Can you work these out from the model? Positions are in its coordinate system, mm. A direction names the side the tool comes from. Coordinates: 2 decimals unless noted, no trailing zeros. Loops run counter-clockwise (first coordinate to the right, second up) from the corner with the lowest first, then second, coordinate; pieces in that order, holes last. Notation, with made-up numbers: (-15, 53.5) -> (22, 53.5) arc R4 cw to (22, 58.5) -> close; hole circle Ø5 at (78.25, -26.75). An arc over 180 degrees is marked (long way). Use one line per item in the form item = value. Start each with the question number.
(1) I'm going to push flat-ended pins straight in: pin 1 (17 mm diameter, centred on x = 60, y = 50.5, fed in from +Z); pin 2 (3 mm diameter, centred on x = 55, y = 30.5, fed in from +Z); pin 3 (1 mm diameter, centred on y = 39.5, z = 3, fed in from -X); pin 4 (0.9 mm diameter, centred on y = 35.5, z = 2.5, fed in from +X). Where does each tip first touch, or does it pass through?
(2) On a 3-axis mill with a long thin cutter (end or side, diameter ignored), from which of +Z, -Z, +X, -X, +Y, -Y can I reach the whole of each face in a straight line? I mean faces 1 (the flat face through (31.483, 58, 1)), 2 (the flat face through (94.183, 40, 3)), 3 (the flat face through (63.267, 43.688, 2.521)), 4 (the flat face through (31.483, 39, 3)). Say none if no direction works.
(3) Imagine slicing it at A-A (y = 62.5). List the corners of the cut face in (x, z) for me, plus the area to 3 significant figures.
(4) Imagine slicing it at D-D (y = 18.5). List the corners of the cut face in (x, z) for me.
(5) Imagine slicing it at B-B (x = 87.5). List the corners of the cut face in (y, z) for me.
(6) Imagine slicing it at C-C (z = 3.3). List the corners of the cut face in (x, y) for me, plus the area to 3 significant figures.
(7) I need wall thicknesses on line 1 (Y direction, x = 70, z = 0.8); line 2 (Y direction, x = 55, z = 1.4); line 3 (X direction, y = 48, z = 1.55). Which ranges of each line are inside material? Lowest first, please. Write a range as [from, to].
(8) Thinking about a two-plate mould opening in Y: for faces 5 (the flat face through (62, 68.292, 1)), 6 (the flat face through (96.083, 40, 1)), 7 (the flat face through (62.4, 66.392, 1.2)), which applies, released by +Y, released by -Y, zero draft, split by the parting line, or undercut?
Autodesk Fusion 360 part; units mm, degrees
sketch "Schizzo1" plane through (0, 0, 0) normal (0, 0, 1) x (1, 0, 0)
  line L0 (29.4832, 68.3919) -> (96.1832, 68.3919) construction
  line L1 (96.1832, 68.3919) -> (96.1832, 10.6919) construction
  line L2 (96.1832, 10.6919) -> (29.4832, 10.6919) construction
  line L3 (29.4832, 10.6919) -> (29.4832, 68.3919) construction
  line L4 (96.0832, 10.7919) -> (29.5832, 10.7919)
  line L5 (29.5832, 10.7919) -> (29.5832, 68.2919)
  line L6 (29.5832, 68.2919) -> (96.0832, 68.2919)
  line L7 (96.0832, 68.2919) -> (96.0832, 10.7919)
  line L8 (94.1832, 12.6919) -> (31.4832, 12.6919)
  line L9 (31.4832, 12.6919) -> (31.4832, 66.3919)
  line L10 (31.4832, 66.3919) -> (94.1832, 66.3919)
  line L11 (94.1832, 66.3919) -> (94.1832, 12.6919)
  line L12 (31.4832, 66.3919) -> (57.4832, 66.3919)
  line L13 (57.4832, 66.3919) -> (57.4832, 56.3919)
  line L14 (57.4832, 56.3919) -> (31.4832, 56.3919)
  line L15 (31.4832, 56.3919) -> (31.4832, 66.3919)
  line L16 (65.4832, 66.3919) -> (91.4832, 66.3919)
  line L17 (91.4832, 56.3919) -> (65.4832, 56.3919)
  line L18 (91.4832, 66.3919) -> (91.4832, 56.3919)
  line L19 (65.4832, 56.3919) -> (65.4832, 66.3919)
  line L20 (29.4832, 39.5419) -> (96.1832, 39.5419) construction
  line L21 (31.4832, 44.5419) -> (94.1832, 44.5419)
  line L22 (31.4832, 34.5419) -> (94.1832, 34.5419)
  line L23 (62.8332, 68.3919) -> (62.8332, 10.7919) construction
  dimension "d1" = 66.7
  dimension "d2" = 57.7
  dimension "d3" = 0.1
  dimension "d4" = 2
  dimension "d5" = 26
  dimension "d6" = 10
  dimension "d9" = 34
  dimension "d10" = 0
  dimension "d16" = 10
extrude "Estrusione1" add sketch "Schizzo1" along normal blind 1 contours L8 L9 L11 L22 | L9 L11 L21 L22 | L9 L10 L11 L13 L14 L17 L18 L19 L21
extrude "Estrusione2" add sketch "Schizzo1" along normal blind 2
fillet "Raccordo1" radius 2 4 edges at (29.5832, 10.7919, 1) (96.0832, 10.7919, 1) (96.0832, 68.2919, 1) (29.5832, 68.2919, 1)
extrude "Estrusione3" add sketch "Schizzo1" along normal blind 4 contours L9 L11 L21 L22
ref_plane "Piano di lavoro1" through (62.8332, 39.5919, 0) normal (-1, 0, 0) x (0, -1, 0)
sketch "Schizzo2" plane through (62.8332, 0, 0) normal (-1, 0, 0) x (0, -1, 0)
  line L0 (-34.5419, 1) -> (-44.5419, 1) construction
  line L1 (-34.5419, 1) -> (-34.5419, 4)
  line L2 (-34.5419, 4) -> (-36.274, 1)
  line L3 (-36.274, 1) -> (-34.5419, 1)
  line L4 (-39.5419, 1) -> (-39.5419, 4) construction
  line L5 (-44.5419, 4) -> (-34.5419, 4) construction
  line L6 (-44.5419, 4) -> (-42.8099, 1)
  line L7 (-42.8099, 1) -> (-44.5419, 1)
  line L8 (-44.5419, 1) -> (-44.5419, 4)
  point P0 (-34.5419, 1)
  point P1 (-44.5419, 1)
  dimension "d20" = 30
extrude "Estrusione4" cut sketch "Schizzo2" along normal mid plane 62
Worked out:
q1.pin_1 = 4
q1.pin_2 = 1
q1.pin_3 = 31.48
q1.pin_4 = 94.18
q2.face_1 = +Z
q2.face_2 = +Z, +X, +Y, -Y
q2.face_3 = none
q2.face_4 = +Z, -X, +Y, -Y
q3.outline = (29.58, 0) -> (31.48, 0) -> (31.48, 2) -> (29.58, 2) -> close; (57.48, 0) -> (65.48, 0) -> (65.48, 1) -> (57.48, 1) -> close; (91.48, 0) -> (96.08, 0) -> (96.08, 2) -> (94.18, 2) -> (94.18, 1) -> (91.48, 1) -> close
q3.area = 18.3 mm2
q4.outline = (29.58, 0) -> (96.08, 0) -> (96.08, 2) -> (94.18, 2) -> (94.18, 1) -> (31.48, 1) -> (31.48, 2) -> (29.58, 2) -> close
q5.outline = (10.79, 0) -> (56.39, 0) -> (56.39, 1) -> (42.81, 1) -> (44.54, 4) -> (34.54, 4) -> (36.27, 1) -> (12.69, 1) -> (12.69, 2) -> (10.79, 2) -> close; (66.39, 0) -> (68.29, 0) -> (68.29, 2) -> (66.39, 2) -> close
q6.outline = (31.48, 34.54) -> (31.83, 34.54) -> (31.83, 34.95) -> (93.83, 34.95) -> (93.83, 34.54) -> (94.18, 34.54) -> (94.18, 44.54) -> (93.83, 44.54) -> (93.83, 44.14) -> (31.83, 44.14) -> (31.83, 44.54) -> (31.48, 44.54) -> close
q6.area = 577 mm2
q7.line_1 = [10.79, 56.39], [66.39, 68.29]
q7.line_2 = [10.79, 12.69], [36.04, 43.04], [66.39, 68.29]
q7.line_3 = [29.58, 31.48], [94.18, 96.08]
q8.face_5 = released by +Y
q8.face_6 = zero draft
q8.face_7 = undercut
